Source: CAD feature listing. Evaluate the final solid. Frame: model axes, mm. A direction names the side the tool comes from. Round coordinates to 2 decimals unless told otherwise and drop trailing zeros. Order: outer loops, then holes, each group sorted by start corner. A loop starts at its lowest first (then second) coordinate and runs counter-clockwise, first axis right, second up. Notation, with made-up numbers: M 85.5,-17.5 L 99.5,-17.5 A15 ccw 99.5,3.5 Z; hole C 53.25,44 d2. An arc over 180 degrees is marked long. Use one line per item in the form item = value. Start each with the question number.
Q1. Section A-A (x = 64). Return the cut outline in (y, z) (3 decimals), plus the area to 3 significant figures.
Q2. Section B-B (z = -127). Give the number of separate pieces and of enclosed holes in the cut face, plus the area to 3 significant figures.
Q3. Contact query for flat-ended pins moving along their axis: pin 1 (6.5 mm diameter, centred on x = 73.12, z = -70.75, fed in from -Y); pin 2 (19 mm diameter, centred on x = 127, z = -127, fed in from -Y); pin 3 (8.5 mm diameter, centred on x = 113.37, z = -134.38, fed in from +Y) (3 decimals); pin 4 (4 mm diameter, centred on x = 184, y = 11, fed in from -Z). Output: stop coordinate, or through.
Q4. Material intervals for probe 1 along Z at (x, y) = (125.5, 4); probe 2 along X at (y, z) = (8.5, -72.5); probe 3 along Z at (x, y) = (56, 12.25), sorted ascending.
Q5. Section D-D (x = 173). Return the cut outline in (y, z), plus the area to 3 significant figures.
Q6. Pull-direction query (Z, two-part tool) for faces 1 (the cylindrical face through (130.31, 4.88, -110.01)), 2 (the flat face through (127, 9, 0)), 3 (the flat face through (127, 9, -254)); classes: pulls with the +Z half, pulls with the -Z half, needs draft (parallel to the pull), parting line crosses it, or undercut.
Q7. Reachability of faces 4 (the cylindrical face through (107.846, 4.696, -40.33)), 5 (the cylindrical face through (134.629, 14.354, -102.773)) from +Z, -Z, +X, -X, +Y, -Y: full face, straight path, thin tool, end or side. Return the list, or none.
from build123d import *

# Parameters (mm, degrees)
SKETCH1_W                                         = 254
SKETCH1_H                                         = 254
BOSS_EXTRUDE1_DEPTH                               = 19.05
SKETCH2_R                                         = 25.4
CUT_EXTRUDE1_DEPTH                                = 9.525
SKETCH3_R                                         = 5.999999938
CUT_EXTRUDE2_DEPTH                                = 360.336507504
CBORE_FOR_M3_SHCS1_AT_2_COUNT                     = 2
CBORE_FOR_M3_SHCS1_AT_2_PITCH                     = 15.5
CBORE_FOR_M3_SHCS1_AT_3_COUNT                     = 2
CBORE_FOR_M3_SHCS1_AT_3_PITCH                     = 26.846787517
CBORE_FOR_M3_SHCS1_AT_4_COUNT                     = 2
CBORE_FOR_M3_SHCS1_AT_4_PITCH                     = 31
CBORE_FOR_M3_SHCS1_AT_5_COUNT                     = 2
CBORE_FOR_M3_SHCS1_AT_5_PITCH                     = 26.846787517
CBORE_FOR_M3_SHCS1_AT_6_COUNT                     = 2
CBORE_FOR_M3_SHCS1_AT_6_PITCH                     = 15.5
SKETCH6_R                                         = 19.05
CUT_EXTRUDE3_DEPTH                                = 2.54
SKETCH7_R                                         = 19.05
CUT_EXTRUDE4_DEPTH                                = 2.54
FILLET1_SIZE                                      = 107.95
CSK_FOR_8_FLAT_HEAD_MACHINE_SCREW_100_D           = 4.9149
CSK_FOR_8_FLAT_HEAD_MACHINE_SCREW_100_CSINK_D     = 8.4328
CSK_FOR_8_FLAT_HEAD_MACHINE_SCREW_100_CSINK_ANGLE = 100
CUT_EXTRUDE6_DEPTH                                = 360.412804759
CUT_EXTRUDE6_DEPTH_BACK                           = 360.412804759
SKETCH14_R                                        = 21.59


with BuildPart() as part:
    # Sketch1 → Boss-Extrude1 (new body)
    with BuildSketch(Plane(origin=(0, 0, 0), x_dir=(1, 0, 0), z_dir=(0, 1, 0))):
        with Locations((127, 127)):
            Rectangle(SKETCH1_W, SKETCH1_H)
    extrude(amount=BOSS_EXTRUDE1_DEPTH)

    # Sketch2 → Cut-Extrude1 (cut)
    with BuildSketch(Plane(origin=(0, 19.05, 0), x_dir=(1, 0, 0), z_dir=(0, 1, 0))):
        with Locations(Location((50.292, 127, 0), (0, 0, 270))):
            Circle(SKETCH2_R)
        with Locations(Location((127, 50.292, 0), (0, 0, 270))):
            Circle(SKETCH2_R)
        with Locations(Location((127, 127, 0), (0, 0, 270))):
            Circle(SKETCH2_R)
        with Locations(Location((203.708, 127, 0), (0, 0, 270))):
            Circle(SKETCH2_R)
        with Locations(Location((127, 203.708, 0), (0, 0, 270))):
            Circle(SKETCH2_R)
    extrude(amount=-CUT_EXTRUDE1_DEPTH, mode=Mode.SUBTRACT)

    # Sketch3 → Cut-Extrude2 (cut, through all)
    with BuildSketch(Plane(origin=(0, 9.525, 0), x_dir=(1, 0, 0), z_dir=(0, 1, 0))):
        with Locations(Location((127, 127, 0), (0, 0, 270))):
            Circle(SKETCH3_R)
    extrude(amount=-CUT_EXTRUDE2_DEPTH, mode=Mode.SUBTRACT)

    # Sketch5 → CBORE for M3 SHCS1 (revolve, cut)
    with BuildSketch(Plane(origin=(127.424882459, 9.525, -111.505824485), x_dir=(0, 0, 1), z_dir=(1, 0, 0))):
        Polygon((0, 0), (0, 11.689463052), (1.7, 10.668), (1.7, 6.81), (3.25, 6.81), (3.25, 0.025), (3.275, 0), align=None)
    cbore_for_m3_shcs1 = revolve(axis=Axis((127.424882459, 15.875, -111.505824485), (0, -1, 0)), mode=Mode.SUBTRACT)

    # CBORE for M3 SHCS1 at 2: CBORE for M3 SHCS1 ×2
    with Locations(*[Vector(-0.8794058604138406, 0, -0.47607282286410013) * (i * CBORE_FOR_M3_SHCS1_AT_2_PITCH) for i in range(1, CBORE_FOR_M3_SHCS1_AT_2_COUNT)]):
        add(cbore_for_m3_shcs1, mode=Mode.SUBTRACT)

    # CBORE for M3 SHCS1 at 3: CBORE for M3 SHCS1 ×2
    with Locations(*[Vector(-0.5235514039232533, 0, -0.8519940888585968) * (i * CBORE_FOR_M3_SHCS1_AT_3_PITCH) for i in range(1, CBORE_FOR_M3_SHCS1_AT_3_COUNT)]):
        add(cbore_for_m3_shcs1, mode=Mode.SUBTRACT)

    # CBORE for M3 SHCS1 at 4: CBORE for M3 SHCS1 ×2
    with Locations(*[Vector(-0.027411771555246985, 0, -0.9996242267873479) * (i * CBORE_FOR_M3_SHCS1_AT_4_PITCH) for i in range(1, CBORE_FOR_M3_SHCS1_AT_4_COUNT)]):
        add(cbore_for_m3_shcs1, mode=Mode.SUBTRACT)

    # CBORE for M3 SHCS1 at 5: CBORE for M3 SHCS1 ×2
    with Locations(*[Vector(0.47607282286409475, 0, -0.8794058604138435) * (i * CBORE_FOR_M3_SHCS1_AT_5_PITCH) for i in range(1, CBORE_FOR_M3_SHCS1_AT_5_COUNT)]):
        add(cbore_for_m3_shcs1, mode=Mode.SUBTRACT)

    # CBORE for M3 SHCS1 at 6: CBORE for M3 SHCS1 ×2
    with Locations(*[Vector(0.8519940888585981, 0, -0.5235514039232514) * (i * CBORE_FOR_M3_SHCS1_AT_6_PITCH) for i in range(1, CBORE_FOR_M3_SHCS1_AT_6_COUNT)]):
        add(cbore_for_m3_shcs1, mode=Mode.SUBTRACT)

    # Sketch6 → Cut-Extrude3 (cut)
    with BuildSketch(Plane(origin=(0, 9.525, 0), x_dir=(1, 0, 0), z_dir=(0, 1, 0))):
        with Locations(Location((127, 50.292, 0), (0, 0, 270))):
            Circle(SKETCH6_R)
        with Locations(Location((50.546, 127.254, 0), (0, 0, 270))):
            Circle(SKETCH6_R)
        with Locations(Location((127.508, 203.708, 0), (0, 0, 270))):
            Circle(SKETCH6_R)
        with Locations(Location((203.962, 126.746, 0), (0, 0, 270))):
            Circle(SKETCH6_R)
    extrude(amount=-CUT_EXTRUDE3_DEPTH, mode=Mode.SUBTRACT)

    # Sketch7 → Cut-Extrude4 (cut)
    with BuildSketch(Plane(origin=(0, 9.525, 0), x_dir=(1, 0, 0), z_dir=(0, 1, 0))):
        with Locations(Location((127, 127, 0), (0, 0, 270))):
            Circle(SKETCH7_R)
    extrude(amount=-CUT_EXTRUDE4_DEPTH, mode=Mode.SUBTRACT)

    # Fillet1
    fillet1_edges = [part.edges().sort_by_distance(p)[0] for p in [
        (0, 9.525, -254),
        (254, 9.525, -254),
        (254, 9.525, 0),
        (0, 9.525, 0),
    ]]
    chamfer(fillet1_edges, length=FILLET1_SIZE)

    # CSK for #8 Flat Head Machine Screw (100)2 (through all)
    with Locations(Plane(origin=(0, 0, 0), x_dir=(-1, 0, 0), z_dir=(0, -1, 0))):
        with Locations((-183.247438789, 73.118463274), (-73.118463274, 70.752561211), (-183.247438789, 180.881536726), (-73.118463274, 183.247438789)):
            CounterSinkHole(CSK_FOR_8_FLAT_HEAD_MACHINE_SCREW_100_D / 2, CSK_FOR_8_FLAT_HEAD_MACHINE_SCREW_100_CSINK_D / 2, counter_sink_angle=CSK_FOR_8_FLAT_HEAD_MACHINE_SCREW_100_CSINK_ANGLE)

    # Sketch14 → Cut-Extrude6 (cut, two sides: drawn at the far end of the back side and taken through both)
    with BuildSketch(Plane(origin=(0, 6.985, 0), x_dir=(1, 0, 0), z_dir=(0, 1, 0)).offset(-CUT_EXTRUDE6_DEPTH_BACK)):
        with Locations(Location((127, 50.292, 0), (0, 0, 270))):
            Circle(SKETCH14_R)
        with Locations(Location((203.962, 126.746, 0), (0, 0, 270))):
            Circle(SKETCH14_R)
        with Locations(Location((127.508, 203.708, 0), (0, 0, 270))):
            Circle(SKETCH14_R)
        with Locations(Location((50.546, 127.254, 0), (0, 0, 270))):
            Circle(SKETCH14_R)
    extrude(amount=CUT_EXTRUDE6_DEPTH + CUT_EXTRUDE6_DEPTH_BACK, mode=Mode.SUBTRACT)


solid = part.part
Results list:
q1.outline = M 0,-210.05 L 19.05,-210.05 L 19.05,-148.383 L 9.525,-148.383 L 9.525,-144.139 L 0,-144.139 Z; M 0,-110.369 L 9.525,-110.369 L 9.525,-105.617 L 19.05,-105.617 L 19.05,-43.95 L 0,-43.95 Z
q1.area = 2,440 mm2
q2.separate_pieces = 4
q2.enclosed_holes = 0
q2.area = 2,380 mm2
q3.pin_1 = 0.81
q3.pin_2 = 0
q3.pin_3 = 9.525
q3.pin_4 = -218.05
q4.probe_1 = -254 to -225.2, -182.21 to -145.56, -139.43 to -132.81, -121.19 to -114.12, -108.89 to -71.83, -28.75 to 0
q4.probe_2 = 35.45 to 71.39, 74.85 to 180.87, 185.63 to 218.55
q4.probe_3 = -202.05 to -151.75, -102.25 to -51.95
q5.outline = M 0,-227.05 L 19.05,-227.05 L 19.05,-26.95 L 0,-26.95 Z
q5.area = 3,810 mm2
q6.face_1 = undercut
q6.face_2 = pulls with the +Z half
q6.face_3 = pulls with the -Z half
q7.face_4 = +Y, -Y
q7.face_5 = +Y
